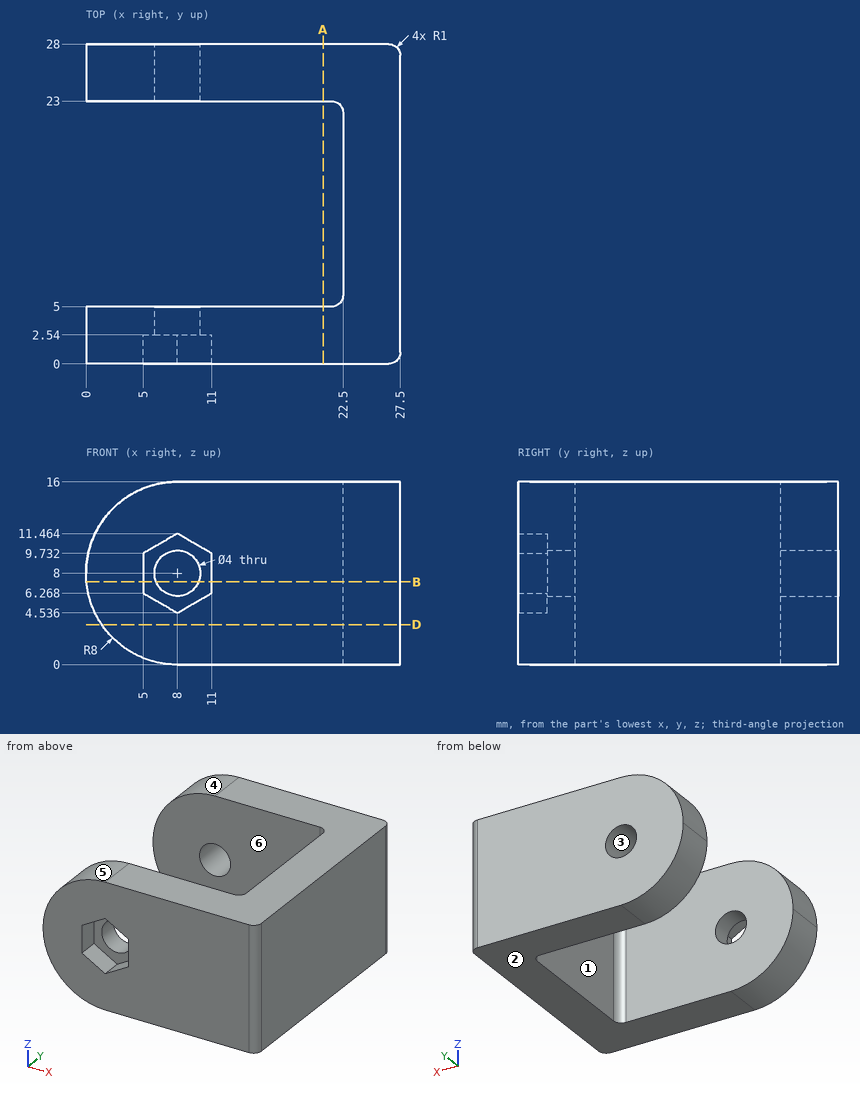
The figure shows three views and two pictorial views of one solid part (mm, origin at its lowest corner). Answer the questions. A direction names the side the tool comes from. Give positions to 0.01 mm unless a question says otherwise; leave off trailing zeros. Write each loop counter-clockwise with the first axis right and the second up, starting at its lowest first coordinate (ties: lowest second). Pieces come first, ordered by that corner, then holes. Notation, with made-up numbers: (16, 26.5) - (38, 26.5) arc R30 cw to (38, 65.5) - close; hole circle Ø5 at (60, 41). An arc over 180 degrees is marked (long way). Return JSON: item names as keys, results as strings.
Q1. For the marked faces 5 and 6, determine the directions among +Z, -Z, +X, -X, +Y, -Y from which every point of the face is accessible in a straight line to the end or side of a thin tool.
Reply:
{"face 5": "+Z, -X, +Y, -Y", "face 6": "+Z, -Z, -X"}
Q2. A cutting plane is placed at D-D, the plane z = 3.5. Determine the outline of the cut face in (x, y).
Reply:
{"outline": "(1.39, 0) - (26.5, 0) arc R1 ccw to (27.5, 1) - (27.5, 27) arc R1 ccw to (26.5, 28) - (1.39, 28) - (1.39, 23) - (21.5, 23) arc R1 cw to (22.5, 22) - (22.5, 6) arc R1 cw to (21.5, 5) - (1.39, 5) - close"}
Q3. A cutting plane is placed at A-A, the plane x = 20.75. Determine the outline of the cut face in (y, z), and give its area (3 significant figures).
Reply:
{"outline": "(0, 0) - (5, 0) - (5, 16) - (0, 16) - close; (23, 0) - (28, 0) - (28, 16) - (23, 16) - close", "area": "160 mm²"}
Q4. Given P1, Ø2, axis at y = 16, z = 5, coming from the -X side, flat-ended and moving along its own axis, determine where the tip first touches the part or whether it passes through.
Reply:
{"P1": "x = 22.5"}
Q5. For a pull along Z with two mould halves and no side action, classify the marked faces 1, 2, 3 and 4 as released by +Z, released by -Z, zero draft, split by the parting line, or undercut.
Reply:
{"face 1": "zero draft", "face 2": "released by -Z", "face 3": "undercut", "face 4": "released by +Z"}
Q6. A cutting plane is placed at B-B, the plane z = 7.25. Determine the outline of the cut face in (x, y).
Reply:
{"outline": "(0.04, 0) - (5, 0) - (5, 2.54) - (6.15, 2.54) - (6.15, 5) - (0.04, 5) - close; (0.04, 23) - (6.15, 23) - (6.15, 28) - (0.04, 28) - close; (9.85, 2.54) - (11, 2.54) - (11, 0) - (26.5, 0) arc R1 ccw to (27.5, 1) - (27.5, 27) arc R1 ccw to (26.5, 28) - (9.85, 28) - (9.85, 23) - (21.5, 23) arc R1 cw to (22.5, 22) - (22.5, 6) arc R1 cw to (21.5, 5) - (9.85, 5) - close"}
Q7. Consider line 1 along Z through (x, y) = (8, 24.75); line 2 along Y through (x, z) = (16.25, 7.75); line 3 along Y through (x, z) = (8.75, 11). Determine where each line is inside the solid, lowest interval first. Write a range as [from, to].
Reply:
{"line 1": "[0, 6], [10, 16]", "line 2": "[0, 5], [23, 28]", "line 3": "[2.54, 5], [23, 28]"}
